from build123d import *

# Parameters (mm, degrees)
SKETCH1_R           = 1.8
SKETCH1_R_2         = 12
BOSS_EXTRUDE1_DEPTH = 10
SKETCH2_W           = 15
SKETCH2_H           = 28
BOSS_EXTRUDE2_DEPTH = 25
SKETCH3_R           = 2.8
CUT_EXTRUDE1_DEPTH  = 75.813100457
SKETCH4_R           = 4.3
CUT_EXTRUDE2_DEPTH  = 6
FILLET1_R           = 2


with BuildPart() as part:
    # Sketch1 → Boss-Extrude1 (new body)
    with BuildSketch(Plane(origin=(0, 0, 0), x_dir=(1, 0, 0), z_dir=(0, 1, 0))):
        with BuildLine():
            Line((48, 0), (0, 0))
            Line((0, 0), (0, -35.65))
            Line((0, -35.65), (2.031373033, -35.65))
            ThreePointArc((2.031373033, -35.65), (6.25049165, -32.157850963), (10, -36.15))
            ThreePointArc((10, -36.15), (6.25049165, -40.142149037), (2.031373033, -36.65))
            Line((2.031373033, -36.65), (0, -36.65))
            Line((0, -36.65), (0, -58))
            Line((0, -58), (48, -58))
            Line((48, -58), (48, 0))
        make_face()
        with Locations(Location((9.5, -51.65, 0), (0, 0, 270))):
            Circle(SKETCH1_R, mode=Mode.SUBTRACT)
        with Locations(Location((40.5, -51.65, 0), (0, 0, 270))):
            Circle(SKETCH1_R, mode=Mode.SUBTRACT)
        with Locations(Location((25, -36.15, 0), (0, 0, 270))):
            Circle(SKETCH1_R_2, mode=Mode.SUBTRACT)
        with Locations(Location((9.5, -20.65, 0), (0, 0, 270))):
            Circle(SKETCH1_R, mode=Mode.SUBTRACT)
        with Locations(Location((40.5, -20.65, 0), (0, 0, 270))):
            Circle(SKETCH1_R, mode=Mode.SUBTRACT)
    extrude(amount=BOSS_EXTRUDE1_DEPTH)

    # Sketch2 → Boss-Extrude2 (add)
    with BuildSketch(Plane(origin=(0, 0, 0), x_dir=(0, 0, -1), z_dir=(1, 0, 0))):
        with Locations((-7.5, 24)):
            Rectangle(SKETCH2_W, SKETCH2_H)
    extrude(amount=BOSS_EXTRUDE2_DEPTH)

    # Sketch3 → Cut-Extrude1 (cut, through all)
    with BuildSketch(Plane.XY.offset(15)):
        with Locations((6.5, 29.196152423)):
            Circle(SKETCH3_R)
        with Locations((18.5, 29.196152423)):
            Circle(SKETCH3_R)
        with Locations((12.5, 18.803847577)):
            Circle(SKETCH3_R)
    extrude(amount=-CUT_EXTRUDE1_DEPTH, mode=Mode.SUBTRACT)

    # Sketch4 → Cut-Extrude2 (cut)
    with BuildSketch(Plane.XY.offset(15)):
        with Locations((6.5, 29.196152423)):
            Circle(SKETCH4_R)
        with Locations((18.5, 29.196152423)):
            Circle(SKETCH4_R)
        with Locations((12.5, 18.803847577)):
            Circle(SKETCH4_R)
    extrude(amount=-CUT_EXTRUDE2_DEPTH, mode=Mode.SUBTRACT)

    # Fillet1
    fillet1_edges = [part.edges().sort_by_distance(p)[0] for p in [
        (0, 10, 47.325),
        (24, 10, 58),
        (48, 5, 58),
        (0, 5, 58),
        (48, 10, 29),
        (0, 10, 25.325),
        (0, 38, 7.5),
        (0, 24, 15),
        (25, 38, 7.5),
        (25, 24, 15),
    ]]
    fillet(fillet1_edges, radius=FILLET1_R)


solid = part.part
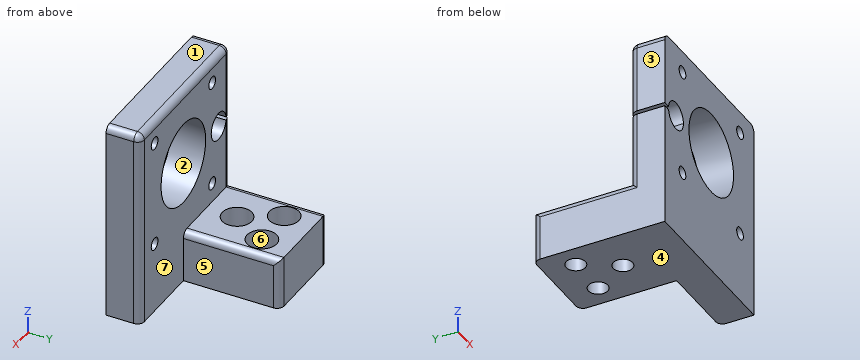
Verification items for the finished model (mm, model axes). Face numbers are marked on the shaded views. A direction names the side the tool comes from. Coordinates: 2 decimals unless noted, no trailing zeros. Write each loop counter-clockwise with the first axis right and the second up, starting at its lowest first coordinate (ties: lowest second). Pieces come first, ordered by that corner, then holes. Notation, with made-up numbers: (-7.75, 75) -> (9.25, 75) arc R30 ccw to (9.25, 101) -> close; hole circle Ø2 at (33.5, -31). An arc over 180 degrees is marked (long way). One line per item, written item: value. Start each with the question number.
Q1. Cross-section at A-A on y = 3. Enter the section's corners in (x, z).
Q2. Access from +Z, -Z, +X, -X, +Y, -Y to the whole of each face (thin tool, end or side, straight path). Record for the marked faces 5, 6 and 7.
Q3. Cross-section at C-C on z = 6.5. Enter the section's corners in (x, y), and give its area (3 significant figures).
Q4. Cross-section at D-D on z = 17.5. Enter the section's corners in (x, y), and give its area (3 significant figures).
Q5. Go/stop test with flat-tipped pins: P1, Ø0.6, axis at x = 1.5, y = 4.5, coming from the +Z side; P2, Ø10.5, axis at x = 13.5, y = 27, coming from the +Z side; P3, Ø21.5, axis at x = 25, z = 36.15, coming from the +Y side; P4, Ø4.5, axis at x = 40.5, z = 51.65, coming from the +Y side. Record where each tip stops, or that it passes through.
Q6. Mould release check, pull along Z, two halves, no side actions. Record for the marked faces 1, 2, 3 and 4: pulls with the +Z half, pulls with the -Z half, needs draft (parallel to the pull), parting line crosses it, or undercut.
Q7. Thickness scan on L1, parallel to X at y = 5, z = 20.65; L2, parallel to Y at x = 6.5, z = 13.1; L3, parallel to X at y = 8, z = 36. Record the ranges inside material, lowest first. Write a range as from..to.
Q8. Cross-section at B-B on x = 6.5. Enter the section's corners in (y, z).
Checked values:
1. outline: (0, 0) -> (48, 0) -> (48, 56) arc R2 ccw to (46, 58) -> (2, 58) arc R2 ccw to (0, 56) -> (0, 36.65) -> (2.03, 36.65) arc R4 cw (long way) to (2.03, 35.65) -> (0, 35.65) -> close; hole circle Ø3.6 at (9.5, 20.65); hole circle Ø3.6 at (9.5, 51.65); hole circle Ø24 at (25, 36.15); hole circle Ø3.6 at (40.5, 20.65); hole circle Ø3.6 at (40.5, 51.65)
2. face 5: +Z, -Z, +X, +Y
2. face 6: +Z
2. face 7: +Z, +X, +Y
3. outline: (0, 0) -> (48, 0) -> (48, 8) arc R2 ccw to (46, 10) -> (25, 10) -> (25, 36) arc R2 ccw to (23, 38) -> (2, 38) arc R2 ccw to (0, 36) -> close; hole circle Ø5.6 at (6.5, 29.2); hole circle Ø5.6 at (12.5, 18.8); hole circle Ø5.6 at (18.5, 29.2)
3. area: 1,100 mm²
4. outline: (0, 0) -> (48, 0) -> (48, 8) arc R2 ccw to (46, 10) -> (2, 10) arc R2 ccw to (0, 8) -> close
4. area: 478 mm²
5. P1: stops at z = 57.99
5. P2: stops at z = 15
5. P3: passes through
5. P4: stops at y = 10
6. face 1: pulls with the +Z half
6. face 2: undercut
6. face 3: needs draft
6. face 4: pulls with the -Z half
7. L1: x = 0..7.7, 11.3..38.7, 42.3..48
7. L2: y = 0..24.9, 33.5..38
7. L3: x = 10..13, 37..48
8. outline: (0, 0) -> (26.4, 0) -> (26.4, 9) -> (24.9, 9) -> (24.9, 15) -> (10, 15) -> (10, 32.18) -> (0, 32.18) -> close; (0, 40.12) -> (10, 40.12) -> (10, 56) arc R2 ccw to (8, 58) -> (0, 58) -> close; (32, 0) -> (38, 0) -> (38, 15) -> (33.5, 15) -> (33.5, 9) -> (32, 9) -> close
